Input: part model. Units: mm. Frame: model coordinates. Face numbers are marked on the shaded views. Coordinates: 2 decimals unless noted, no trailing zeros. Write each loop counter-clockwise with the first axis right and the second up, starting at its lowest first coordinate (ties: lowest second). Pieces come first, ordered by that corner, then holes. Notation, with made-up numbers: (33, 77.5) - (38, 77.5) arc R10 cw to (38, 88.5) - close; hole circle Ø11 at (4.25, 85). An arc over 180 degrees is marked (long way). Use CSV: the item, a comma, the result in double quotes.
```python
from build123d import *

# Parameters (mm, degrees)
F0_R     = 20
F1_DEPTH = 60
F2_R     = 12.5
F3_DEPTH = 20
F4_DEPTH = 20
F5_DEPTH = 20


with BuildPart() as f1:
    # F0 (on Front) → F1 (new body, symmetric)
    with BuildSketch(Plane.XZ):
        Circle(F0_R)
    extrude(amount=F1_DEPTH, both=True)

    # F2 (on Right) → F3 (cut, symmetric)
    with BuildSketch(Plane.YZ):
        Circle(F2_R)
    extrude(amount=F3_DEPTH, both=True, mode=Mode.SUBTRACT)

    # F4 (cut, symmetric): a face of the model
    f4_faces = [f1.faces().sort_by_distance(p)[0] for p in [
        (0, 60, 0),
    ]]
    extrude(f4_faces, amount=F4_DEPTH, both=True, mode=Mode.SUBTRACT)

    # F5 (cut, symmetric): a face of the model
    f5_faces = [f1.faces().sort_by_distance(p)[0] for p in [
        (0, 40, 0),
    ]]
    extrude(f5_faces, amount=F5_DEPTH, both=True, mode=Mode.SUBTRACT)


solid = f1.part
```
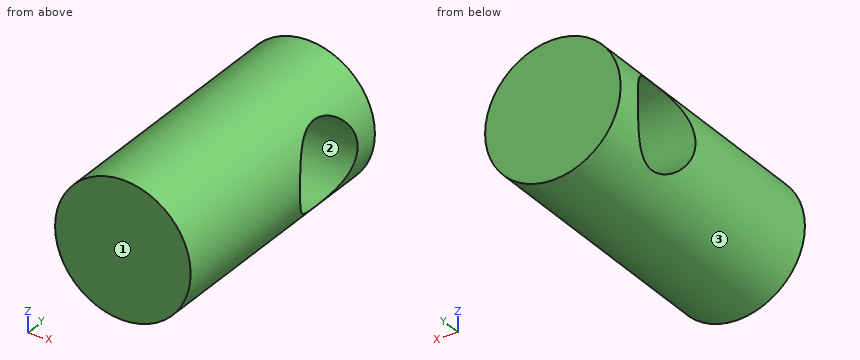
(1) Draft query along Z for the marked faces 1, 2 and 3. Return one class per face: pulls with the +Z half, pulls with the -Z half, needs draft (parallel to the pull), parting line crosses it, or undercut.
Check values:
face 1,"needs draft"
face 2,"undercut"
face 3,"parting line crosses it"
(2) Cut plane A-A on x = 16. Return loops of the section in (y, z).
Check values:
outline,"(-60, -12) - (-3.5, -12) arc R12.5 cw to (-3.5, 12) - (-60, 12) - close; (3.5, -12) - (20, -12) - (20, 12) - (3.5, 12) arc R12.5 cw to start"
(3) Cut plane C-C on x = 0. Return loops of the section in (y, z).
Check values:
outline,"(-60, -20) - (20, -20) - (20, 20) - (-60, 20) - close; hole circle Ø25 at (0, 0)"
(4) Cut plane B-B on z = 0. Return loops of the section in (x, y).
Check values:
outline,"(-20, -60) - (20, -60) - (20, -12.5) - (-20, -12.5) - close; (-20, 12.5) - (20, 12.5) - (20, 20) - (-20, 20) - close"
(5) Pin query (flat end, axial travel): pin 1 Ø1 at (y, z) = (-38.5, -14.5) entering from +X; pin 2 Ø2 at (y, z) = (-28.5, 12.5) entering from -X; pin 3 Ø3 at (x, y) = (-7.5, -49) entering from +Z. Return the tip coordinate at first contact, or that it passes through.
Check values:
pin 1,"x = 14.28"
pin 2,"x = -16.36"
pin 3,"z = 19.08"
(6) Cut plane D-D on y = 0. Return loops of the section in (x, z).
Check values:
outline,"(-15.61, -12.5) arc R20 ccw to (15.61, -12.5) - close; (-15.61, 12.5) - (15.61, 12.5) arc R20 ccw to start"
(7) Ray query, probe 1 along Y at (x, z) = (1, 0); probe 2 along Z at (x, y) = (2, 0); probe 3 along Y at (x, z) = (-12, 2). Return the intervals inside material, ascending. Write a range as from..to.
Check values:
probe 1,"-60..-12.5, 12.5..20"
probe 2,"-19.9..-12.5, 12.5..19.9"
probe 3,"-60..-12.34, 12.34..20"
